Part print with two shaded views. Sizes in mm from the minimum x, y, z corner. A direction names the side the tool comes from. Coordinates: 2 decimals unless noted, no trailing zeros. Order: outer loops, then holes, each group sorted by start corner. A loop starts at its lowest first (then second) coordinate and runs counter-clockwise, first axis right, second up.
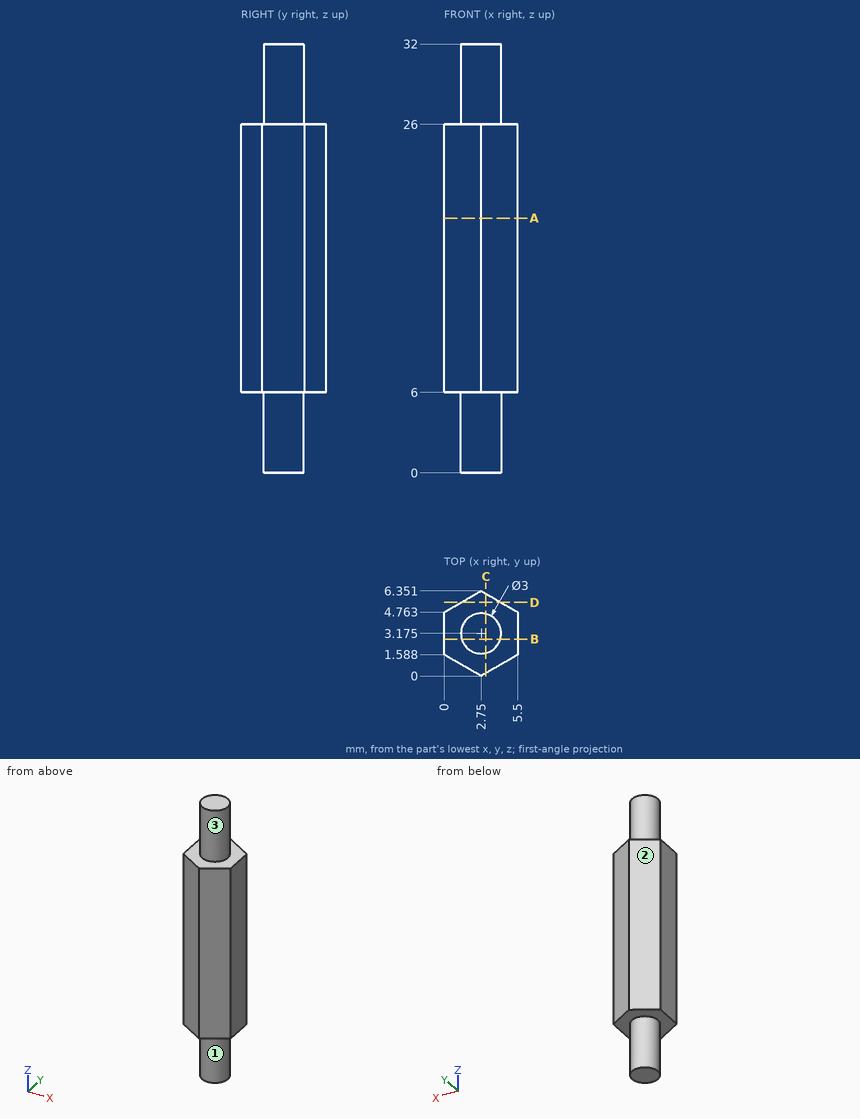
Q1. Cut at C-C on x = 3.1. Write the cut outline in (y, z).
Results list:
outline: (0.2, 6) - (1.72, 6) - (1.72, 0) - (4.63, 0) - (4.63, 6) - (6.15, 6) - (6.15, 26) - (4.63, 26) - (4.63, 32) - (1.72, 32) - (1.72, 26) - (0.2, 26) - close
Q2. Cut at D-D on y = 5.5. Write the cut outline in (x, z).
Results list:
outline: (1.28, 6) - (4.22, 6) - (4.22, 26) - (1.28, 26) - close
Q3. Which spindle directions (+Z, -Z, +X, -X, +Y, -Y) get a long thin tool onto all of the face, cutting with end or side? Do the marked faces 1, 2 and 3. Say none if no direction does.
Results list:
face 1: -Z
face 2: +Z, -Z, -X, +Y
face 3: +Z
Q4. Cut at A-A on z = 19. Write the cut outline in (x, y).
Results list:
outline: (0, 1.59) - (2.75, 0) - (5.5, 1.59) - (5.5, 4.76) - (2.75, 6.35) - (0, 4.76) - close
Q5. Wall check: line 1 along Z through (x, y) = (4.9, 4.25); line 2 along X through (y, z) = (2.5, 2); line 3 along Y through (x, z) = (5.1, 12.5) (1 decimal). Give the ranges that are in metal, low to high.
Results list:
line 1: z = 6 to 26
line 2: x = 1.41 to 4.09
line 3: y = 1.4 to 5
Q6. Cut at B-B on y = 2.75. Write the cut outline in (x, z).
Results list:
outline: (0, 6) - (1.31, 6) - (1.31, 0) - (4.19, 0) - (4.19, 6) - (5.5, 6) - (5.5, 26) - (4.19, 26) - (4.19, 32) - (1.31, 32) - (1.31, 26) - (0, 26) - close
